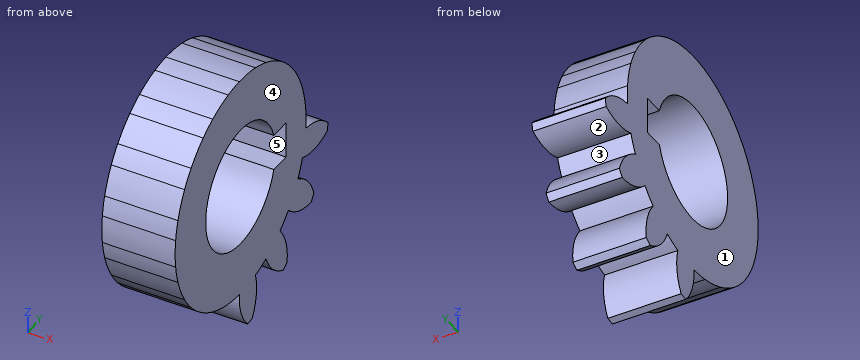
from build123d import *

# Parameters (mm, degrees)
BASPROSKE_W             = 12
BASPROSKE_H             = 25.5
TOOTHCUT_DEPTH          = 39.006578378
TEETHCUTS_COUNT         = 15
TEETHCUTS_ANGLE         = 336
BORSKE_R                = 10
BORE_DEPTH              = 50.0000508
CUT_EXTRUDE1_DEPTH      = 38.954121274
CUT_EXTRUDE2_DEPTH      = 38.669115521
CUT_EXTRUDE2_DEPTH_BACK = 38.669115521
SKETCH3_W               = 6
SKETCH3_H               = 6


with BuildPart() as part:
    # BasProSke → Base-Revolve (revolve)
    with BuildSketch(Plane(origin=(0, 0, 0), x_dir=(1, 0, 0), z_dir=(0, 1, 0)), mode=Mode.PRIVATE) as base_revolve_sk:
        with Locations((6, 12.75)):
            Rectangle(BASPROSKE_W, BASPROSKE_H)
    revolve(base_revolve_sk.sketch.rotate(Axis((-10, 0, 0), (1, 0, 0)), 180), axis=Axis((-10, 0, 0), (1, 0, 0)))

    # TooCutSke → ToothCut (cut, through all)
    with BuildSketch(Plane(origin=(0, 0, 0), x_dir=(0, 0, -1), z_dir=(1, 0, 0))):
        with BuildLine():
            ThreePointArc((1.584594428, 18.681918036), (0, 18.749), (-1.584594428, 18.681918036))
            ThreePointArc((-1.584594428, 18.681918036), (-2.465052499, 22.206073835), (-4.666912141, 25.095138498))
            ThreePointArc((-4.666912141, 25.095138498), (0, 25.5254), (4.666912141, 25.095138498))
            ThreePointArc((4.666912141, 25.095138498), (2.465052499, 22.206073835), (1.584594428, 18.681918036))
        make_face()
    toothcut = extrude(amount=TOOTHCUT_DEPTH, mode=Mode.SUBTRACT)

    # TeethCuts: ToothCut ×15 about axis
    teethcuts_axis = Axis((-10, 0, 0), (1, 0, 0))
    for i in range(1, TEETHCUTS_COUNT):
        add(toothcut.rotate(teethcuts_axis, i * TEETHCUTS_ANGLE / (TEETHCUTS_COUNT - 1)), mode=Mode.SUBTRACT)

    # BorSke → Bore (cut, symmetric)
    with BuildSketch(Plane(origin=(0, 0, 0), x_dir=(0, 0, -1), z_dir=(1, 0, 0))):
        with Locations(Location((0, 0, 0), (0, 0, 180))):
            Circle(BORSKE_R)
    extrude(amount=BORE_DEPTH, both=True, mode=Mode.SUBTRACT)

    # Sketch1 → Cut-Extrude1 (cut, through all)
    with BuildSketch(Plane(origin=(0, 0, 0), x_dir=(0, 0, -1), z_dir=(1, 0, 0))):
        with BuildLine():
            ThreePointArc((18.677788491, -1.632549567), (-13.822692806, -12.667208239), (0, 18.749))
            Line((0, 18.749), (0, 29.219389367))
            Line((0, 29.219389367), (-29.845264735, 29.219389367))
            Line((-29.845264735, 29.219389367), (-29.845264735, -32.484488502))
            Line((-29.845264735, -32.484488502), (30.166423099, -32.484488502))
            Line((30.166423099, -32.484488502), (30.166423099, -1.632549567))
            Line((30.166423099, -1.632549567), (18.677788491, -1.632549567))
        make_face()
    extrude(amount=CUT_EXTRUDE1_DEPTH, mode=Mode.SUBTRACT)

    # Sketch3 → Cut-Extrude2 (cut, two sides: drawn at the far end of the back side and taken through both)
    with BuildSketch(Plane(origin=(0, 0, 0), x_dir=(0, 0, -1), z_dir=(1, 0, 0)).offset(-CUT_EXTRUDE2_DEPTH_BACK)):
        with Locations((0, 10)):
            Rectangle(SKETCH3_W, SKETCH3_H)
    extrude(amount=CUT_EXTRUDE2_DEPTH + CUT_EXTRUDE2_DEPTH_BACK, mode=Mode.SUBTRACT)


solid = part.part
Design review of the part built by this model. Coordinates are the model's own, in mm. Face numbers are marked on the shaded views. A direction names the side the tool comes from. Round coordinates to 2 decimals unless told otherwise and drop trailing zeros. Order: outer loops, then holes, each group sorted by start corner. A loop starts at its lowest first (then second) coordinate and runs counter-clockwise, first axis right, second up.
1) Consider section A-A (y = -1.5). State the section outline as (x, z) points.
The answers:
outline: (0, -18.69) - (12, -18.69) - (12, -9.89) - (0, -9.89) - close; (0, 9.89) - (12, 9.89) - (12, 18.69) - (0, 18.69) - close
2) Consider section B-B (z = 0). State the section outline as (x, y) points.
The answers:
outline: (0, -18.75) - (12, -18.75) - (12, -10) - (0, -10) - close; (0, 13) - (12, 13) - (12, 18.75) - (0, 18.75) - close
3) Machinability: for the marked faces 1 and 2, which of the approach directions +Z, -Z, +X, -X, +Y, -Y give a long, thin tool a straight path to every point of the face, cutting with its end or side? Answer none if there is none.
The answers:
face 1: +Z, -Z, -X, +Y, -Y
face 2: +X, -X
4) Draft analysis for pull direction Z (two halves, no side actions). For the marked faces 3, 4 and 5, state which applies: released by +Z, released by -Z, zero draft, split by the parting line, or undercut.
The answers:
face 3: undercut
face 4: zero draft
face 5: undercut
5) For L1, parallel to Y at x = 6.75, z = -21.5; L2, parallel to Z at x = 7.75, y = 9; L3, parallel to Y at x = 10.5, z = 3.5, list the stretches that pass through material, from the lowest coordinate up.
The answers:
L1: y = -0.12 to 4.56, 10.53 to 13.35
L2: z = -20.13 to -4.36, 4.36 to 16.45
L3: y = -18.42 to -9.37, 9.37 to 18.42
6) Clearance check with flat-ended pins moving along their axes: pin 1 Ø5 at (x, z) = (5.5, 10) entering from +Y; pin 2 Ø10 at (y, z) = (4.5, 1.5) entering from -X; pin 3 Ø4 at (x, y) = (9, 15.5) entering from +Z; pin 4 Ø3 at (x, y) = (5, 11) entering from -Z. State where each tip first meets the part, or that it passes through.
The answers:
pin 1: stops at y = 17.18
pin 2: passes through
pin 3: stops at z = 13.01
pin 4: stops at z = -22.41
